Work out the finished part from the listing and answer in its coordinate system (mm). Face numbers are marked on the shaded views. A direction names the side the tool comes from. Round coordinates to 2 decimals unless told otherwise and drop trailing zeros. Write each loop counter-clockwise with the first axis right and the second up, starting at its lowest first coordinate (ties: lowest second). Pieces come first, ordered by that corner, then holes. Notation, with made-up numbers: M -27.5,20 L -5.5,20 A21 cw -5.5,37 Z; hole C -26,84.25 d1. An arc over 180 degrees is marked long. Answer in a Markdown table with one row per item.
```python
from build123d import *

# Parameters (mm, degrees)
SKETCH1_R           = 2.5
SKETCH1_R_2         = 1.5
BOSS_EXTRUDE1_DEPTH = 5
SKETCH2_W           = 6.4
SKETCH2_H           = 5
BOSS_EXTRUDE2_DEPTH = 13.5
SKETCH3_W           = 2.5
SKETCH3_H           = 5
CUT_EXTRUDE1_DEPTH  = 11.5
SKETCH4_R           = 1.5
CUT_EXTRUDE2_DEPTH  = 7
SKETCH_2_R          = 1.25
CUT_EXTRUDE_1_DEPTH = 10


with BuildPart() as part:
    # Sketch1 → Boss-Extrude1 (new body)
    with BuildSketch(Plane.XY):
        Circle(SKETCH1_R)
        Circle(SKETCH1_R_2, mode=Mode.SUBTRACT)
    extrude(amount=BOSS_EXTRUDE1_DEPTH)

    # Sketch2 → Boss-Extrude2 (add)
    with BuildSketch(Plane.XY.offset(5)):
        Rectangle(SKETCH2_W, SKETCH2_H)
    extrude(amount=BOSS_EXTRUDE2_DEPTH)

    # Sketch3 → Cut-Extrude1 (cut)
    with BuildSketch(Plane.XY.offset(18.5)):
        Rectangle(SKETCH3_W, SKETCH3_H)
    extrude(amount=-CUT_EXTRUDE1_DEPTH, mode=Mode.SUBTRACT)

    # Sketch4 → Cut-Extrude2 (cut)
    with BuildSketch(Plane.ZY.offset(3.2)):
        with Locations((16, 0)):
            Circle(SKETCH4_R)
        with BuildLine():
            Line((16, 2.5), (20, 2.5))
            Line((20, 2.5), (20, -2.5))
            Line((20, -2.5), (16, -2.5))
            ThreePointArc((16, -2.5), (18.5, 0), (16, 2.5))
        make_face()
    extrude(amount=-CUT_EXTRUDE2_DEPTH, mode=Mode.SUBTRACT)

    # 草图2 → 切除-拉伸1 (cut)
    with BuildSketch(Plane(origin=(0, 0, 5), x_dir=(-1, 0, 0), z_dir=(0, 0, -1))):
        Circle(SKETCH_2_R)
    extrude(amount=-CUT_EXTRUDE_1_DEPTH, mode=Mode.SUBTRACT)


solid = part.part
```
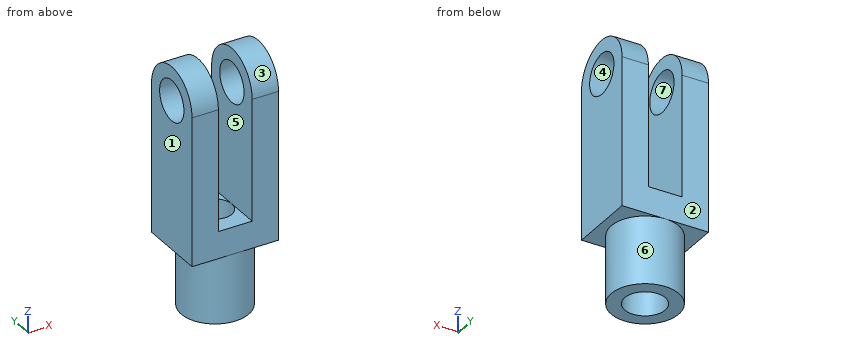
1. The part is cut by section C-C (x = 2.25). Determine the outline of the cut face in (y, z), plus the area to 3 significant figures.
Calculated:
| item | result |
|---|---|
| outline | M -2.5,5 L -1.09,5 L -1.09,0 L 1.09,0 L 1.09,5 L 2.5,5 L 2.5,16 A2.5 ccw -2.5,16 Z; hole C 0,16 d3 |
| area | 68.6 mm² |
2. Consider line 1 along X through (y, z) = (0, 6.15); line 2 along Y through (x, z) = (0, 3.75); line 3 along Y through (x, z) = (-1.75, 16.5). Determine where each line is inside the solid, lowest interval first. Write a range as from..to.
Calculated:
| item | result |
|---|---|
| line 1 | x = -3.2..-1.25, 1.25..3.2 |
| line 2 | y = -2.5..-1.5, 1.5..2.5 |
| line 3 | y = -2.45..-1.41, 1.41..2.45 |
3. The part is cut by section B-B (x = -1). Determine the outline of the cut face in (y, z).
Calculated:
| item | result |
|---|---|
| outline | M -2.5,5 L -2.29,5 L -2.29,0 L -1.12,0 L -1.12,5 L -0.75,5 L -0.75,7 L -2.5,7 Z; M 0.75,5 L 1.12,5 L 1.12,0 L 2.29,0 L 2.29,5 L 2.5,5 L 2.5,7 L 0.75,7 Z |
4. The part is cut by section A-A (z = 9.5). Determine the outline of the cut face in (x, y).
Calculated:
| item | result |
|---|---|
| outline | M -3.2,-2.5 L -1.25,-2.5 L -1.25,2.5 L -3.2,2.5 Z; M 1.25,-2.5 L 3.2,-2.5 L 3.2,2.5 L 1.25,2.5 Z |
5. Given pin 1 (0.8 mm diameter, centred on x = -0.5, y = 1.5, fed in from +Z); pin 2 (1.5 mm diameter, centred on x = 1, y = 2, fed in from +Z); pin 3 (2 mm diameter, centred on x = -0.5, y = -1.5, fed in from +Z), each flat-ended and moving along its own axis, determine where each tip first touches the part or whether it passes through.
Calculated:
| item | result |
|---|---|
| pin 1 | stops at z = 7 |
| pin 2 | stops at z = 18.14 |
| pin 3 | stops at z = 18.36 |
6. A tool of negligible diameter and unlimited length cuts with its end or side. For the marked faces 5, 6 and 7, from which of +Z, -Z, +X, -X, +Y, -Y can it reach the whole face along a straight path? Write none if from no direction.
Calculated:
| item | result |
|---|---|
| face 5 | +Z, +Y, -Y |
| face 6 | -Z |
| face 7 | +X, -X |
7. The part is cut by section D-D (y = 0.35). Determine the outline of the cut face in (x, z), plus the area to 3 significant figures.
Calculated:
| item | result |
|---|---|
| outline | M -3.2,5 L -2.48,5 L -2.48,0 L -1.46,0 L -1.46,5 L -1.2,5 L -1.2,7 L -1.25,7 L -1.25,14.54 L -3.2,14.54 Z; M -3.2,17.46 L -1.25,17.46 L -1.25,18.48 L -3.2,18.48 Z; M 1.2,5 L 1.46,5 L 1.46,0 L 2.48,0 L 2.48,5 L 3.2,5 L 3.2,14.54 L 1.25,14.54 L 1.25,7 L 1.2,7 Z; M 1.25,17.46 L 3.2,17.46 L 3.2,18.48 L 1.25,18.48 Z |
| area | 51.5 mm² |
8. Determine the mould class of the marked faces 1, 2, 3 and 4 for opening direction Y: released by +Y, released by -Y, zero draft, split by the parting line, or undercut.
Calculated:
| item | result |
|---|---|
| face 1 | zero draft |
| face 2 | released by +Y |
| face 3 | split by the parting line |
| face 4 | undercut |
